Source: CAD feature listing. Evaluate the final solid. Frame: model axes, mm. A direction names the side the tool comes from. Give positions to 0.01 mm unless a question says otherwise; leave off trailing zeros. Order: outer loops, then holes, each group sorted by start corner. A loop starts at its lowest first (then second) coordinate and runs counter-clockwise, first axis right, second up.
from build123d import *

# Parameters (mm, degrees)
F0_W     = 580
F0_H     = 248
F0_R     = 5.5
F1_DEPTH = 40
F2_W     = 55
F2_H     = 10
F3_DEPTH = 580.001
F4_SIZE2 = 6
F4_SIZE  = 6


with BuildPart() as f1:
    # F0 (on Top) → F1 (new body)
    with BuildSketch(Plane.XY):
        Rectangle(F0_W, F0_H)
        with Locations((-265, -92)):
            Circle(F0_R, mode=Mode.SUBTRACT)
        with Locations((-132.5, -92)):
            Circle(F0_R, mode=Mode.SUBTRACT)
        with Locations((0, -92)):
            Circle(F0_R, mode=Mode.SUBTRACT)
        with Locations((132.5, -92)):
            Circle(F0_R, mode=Mode.SUBTRACT)
        with Locations((265, -92)):
            Circle(F0_R, mode=Mode.SUBTRACT)
        with Locations((-265, 92)):
            Circle(F0_R, mode=Mode.SUBTRACT)
        with Locations((-132.5, 92)):
            Circle(F0_R, mode=Mode.SUBTRACT)
        with Locations((0, 92)):
            Circle(F0_R, mode=Mode.SUBTRACT)
        with Locations((132.5, 92)):
            Circle(F0_R, mode=Mode.SUBTRACT)
        with Locations((265, 92)):
            Circle(F0_R, mode=Mode.SUBTRACT)
    extrude(amount=F1_DEPTH)

    # F2 (on face) → F3 (cut, through all)
    with BuildSketch(Plane.YZ.offset(290)):
        with Locations((96.5, 5)):
            Rectangle(F2_W, F2_H)
        with Locations((-96.5, 5)):
            Rectangle(F2_W, F2_H)
    extrude(amount=-F3_DEPTH, mode=Mode.SUBTRACT)

    # F4
    f4_edges = [f1.edges().sort_by_distance(p)[0] for p in [
        (259.5, 92, 40),
        (127, 92, 40),
        (259.5, -92, 40),
        (127, -92, 40),
        (-5.5, -92, 40),
        (-5.5, 92, 40),
        (-138, -92, 40),
        (-138, 92, 40),
        (-270.5, 92, 40),
        (-270.5, -92, 40),
    ]]
    chamfer(f4_edges, length=F4_SIZE, length2=F4_SIZE2)


solid = f1.part
1) Ray query, L1, parallel to Y at x = 0, z = 16.25; L2, parallel to X at y = -92, z = 22; L3, parallel to Z at x = -224, y = -86. Return the intervals inside material, ascending.
Checks:
L1: y = -124 to -97.5, -86.5 to 86.5, 97.5 to 124
L2: x = -290 to -270.5, -259.5 to -138, -127 to -5.5, 5.5 to 127, 138 to 259.5, 270.5 to 290
L3: z = 10 to 40
2) Reachability of faces 5 (the face through (128.45, 95.72, 21.83)), 6 (the face through (4, -97, 10)) from +Z, -Z, +X, -X, +Y, -Y: full face, straight path, thin tool, end or side. Return the list, or none.
Checks:
face 5: +Z, -Z
face 6: -Z, +X, -X, -Y
3) Section query A-A on y = 92. State how many separate pieces and enclosed holes the cut face has, and give its area (3 significant figures).
Checks:
separate pieces: 6
enclosed holes: 0
area: 15,600 mm2
4) First-contact query: pin 1 Ø17.5 at (x, y) = (132.5, 92) entering from -Z; pin 2 Ø9 at (x, y) = (265, 92) entering from -Z; pin 3 Ø17.5 at (x, y) = (-265, -92) entering from +Z; pin 4 Ø8 at (x, z) = (-81, 4) entering from +Y. Flat tips, straight axial feed; report the tip coordinate or a pass-through.
Checks:
pin 1: stops at z = 10
pin 2: passes through
pin 3: stops at z = 37.25
pin 4: stops at y = 69
5) Pull-direction query (Y, two-part tool) for faces 1 (the face through (-127.15, 89.78, 34.29)), 2 (the face through (131.24, 86.35, 34.29)), 3 (the face through (-4, 2, 40)), 4 (the face through (4, -69, 5)); classes: +Y half, -Y half, draft (parallel to the pull), parting line (faces both ways), or undercut.
Checks:
face 1: undercut
face 2: undercut
face 3: draft
face 4: -Y half
6) Section query C-C on x = 83. Output: boundary loops of the cut face in (y, z).
Checks:
outline: (-124, 10) - (-69, 10) - (-69, 0) - (69, 0) - (69, 10) - (124, 10) - (124, 40) - (-124, 40) - close
7) Section query B-B on x = 265. Output: boundary loops of the cut face in (y, z), and give its area (3 significant figures).
Checks:
outline: (-124, 10) - (-97.5, 10) - (-97.5, 34) - (-103.5, 40) - (-124, 40) - close; (-86.5, 10) - (-69, 10) - (-69, 0) - (69, 0) - (69, 10) - (86.5, 10) - (86.5, 34) - (80.5, 40) - (-80.5, 40) - (-86.5, 34) - close; (97.5, 10) - (124, 10) - (124, 40) - (103.5, 40) - (97.5, 34) - close
area: 8,090 mm2
